The listing builds one solid part. Answer for the finished solid, in the listing's coordinates (mm). A direction names the side the tool comes from. Round coordinates to 2 decimals unless told otherwise and drop trailing zeros. Write each loop counter-clockwise with the first axis right and the second up, starting at its lowest first coordinate (ties: lowest second). Pieces come first, ordered by that corner, then holes. Notation, with made-up numbers: M 36,34 L 53,34 A32 ccw 53,61 Z; hole C 58,59.25 d6. An arc over 180 degrees is marked long. One line per item, written item: value. Start each with the question number.
(1) Given P1, Ø6, axis at x = 23, y = -94.5, coming from the +Z side; P2, Ø5, axis at x = 13, y = -127, coming from the -Z side, each flat-ended and moving along its own axis, determine where each tip first touches the part or whether it passes through.
(2) Section B-B (y = -90) is taken. Determine the outline of the cut face in (x, z).
(3) Section A-A (z = 14.25) is taken. State how many separate pieces and enclosed holes the cut face has, plus the area to 3 significant figures.
(4) For a pull along X with two mould halves and no side action, classify faces 4 (the flat face through (15, -129, 4.5)), 5 (the flat face through (80, -101, 10)), 6 (the flat face through (-1, -30, 10)) as released by +X, released by -X, zero draft, split by the parting line, or undercut.
(5) Consider probe 1 along Y at (x, z) = (20, 4.5); probe 2 along X at (y, z) = (-153, 14.75); probe 3 along Y at (x, z) = (-20, 17). Determine where each line is inside the solid, lowest interval first.
(6) Section C-C (x = -20) is taken. Determine the outline of the cut face in (y, z).
(7) For faces 1 (the flat face through (-1, -99, 20)), 2 (the flat face through (15, -155, 4.5)), 3 (the cylindrical face through (-15.386, -58.872, 13.591)), determine the directions among +Z, -Z, +X, -X, +Y, -Y from which every point of the face is accessible in a straight line to the end or side of a thin tool.
```python
from build123d import *

# Parameters (mm, degrees)
SKETCH1_W               = 160
SKETCH1_H               = 140
BOSS_EXTRUDE1_DEPTH     = 20
CUT_EXTRUDE1_DEPTH      = 189.944436277
CUT_EXTRUDE1_DEPTH_BACK = 189.944436277
SKETCH2_R               = 6.75
SKETCH3_R               = 10
CUT_EXTRUDE3_DEPTH      = 13
CUT_EXTRUDE4_DEPTH      = 189.944436277
CUT_EXTRUDE4_DEPTH_BACK = 189.944436277
SKETCH4_R               = 2.25
SKETCH5_R               = 4
CUT_EXTRUDE6_DEPTH      = 4.5


with BuildPart() as part:
    # Sketch1 → Boss-Extrude1 (new body)
    with BuildSketch(Plane.XY):
        with Locations((0, -100)):
            Rectangle(SKETCH1_W, SKETCH1_H)
    extrude(amount=BOSS_EXTRUDE1_DEPTH)

    # Sketch2 → Cut-Extrude1 (cut, two sides: drawn at the far end of the back side and taken through both)
    with BuildSketch(Plane.XY.offset(-CUT_EXTRUDE1_DEPTH_BACK)):
        with Locations((-20, -50)):
            Circle(SKETCH2_R)
        with Locations((-20, -90)):
            Circle(SKETCH2_R)
        with Locations((20, -50)):
            Circle(SKETCH2_R)
        with Locations((20, -90)):
            Circle(SKETCH2_R)
    extrude(amount=CUT_EXTRUDE1_DEPTH + CUT_EXTRUDE1_DEPTH_BACK, mode=Mode.SUBTRACT)

    # Sketch3 → Cut-Extrude3 (cut)
    with BuildSketch(Plane.XY.offset(20)):
        with Locations((-20, -50)):
            Circle(SKETCH3_R)
        with Locations((-20, -90)):
            Circle(SKETCH3_R)
        with Locations((20, -50)):
            Circle(SKETCH3_R)
        with Locations((20, -90)):
            Circle(SKETCH3_R)
    extrude(amount=-CUT_EXTRUDE3_DEPTH, mode=Mode.SUBTRACT)

    # Sketch4 → Cut-Extrude4 (cut, two sides: drawn at the far end of the back side and taken through both)
    with BuildSketch(Plane.XY.offset(-CUT_EXTRUDE4_DEPTH_BACK)):
        with Locations((-13, -127)):
            Circle(SKETCH4_R)
        with Locations((-13, -153)):
            Circle(SKETCH4_R)
        with Locations((13, -127)):
            Circle(SKETCH4_R)
        with Locations((13, -153)):
            Circle(SKETCH4_R)
    extrude(amount=CUT_EXTRUDE4_DEPTH + CUT_EXTRUDE4_DEPTH_BACK, mode=Mode.SUBTRACT)

    # Sketch5 → Cut-Extrude6 (cut)
    with BuildSketch(Plane.XY):
        with Locations((-13, -127)):
            Circle(SKETCH5_R)
        with Locations((-13, -153)):
            Circle(SKETCH5_R)
        with Locations((13, -127)):
            Circle(SKETCH5_R)
        with Locations((13, -153)):
            Circle(SKETCH5_R)
    extrude(amount=CUT_EXTRUDE6_DEPTH, mode=Mode.SUBTRACT)


solid = part.part
```
Recorded:
1. P1: stops at z = 7
1. P2: stops at z = 4.5
2. outline: M -80,0 L -26.75,0 L -26.75,7 L -30,7 L -30,20 L -80,20 Z; M -13.25,0 L 13.25,0 L 13.25,7 L 10,7 L 10,20 L -10,20 L -10,7 L -13.25,7 Z; M 26.75,0 L 80,0 L 80,20 L 30,20 L 30,7 L 26.75,7 Z
3. separate pieces: 1
3. enclosed holes: 8
3. area: 21,100 mm2
4. face 4: undercut
4. face 5: released by +X
4. face 6: zero draft
5. probe 1: y = -170 to -96.75, -83.25 to -56.75, -43.25 to -30
5. probe 2: x = -80 to -15.25, -10.75 to 10.75, 15.25 to 80
5. probe 3: y = -170 to -100, -80 to -60, -40 to -30
6. outline: M -170,0 L -96.75,0 L -96.75,7 L -100,7 L -100,20 L -170,20 Z; M -83.25,0 L -56.75,0 L -56.75,7 L -60,7 L -60,20 L -80,20 L -80,7 L -83.25,7 Z; M -43.25,0 L -30,0 L -30,20 L -40,20 L -40,7 L -43.25,7 Z
7. face 1: +Z, +X, -X, +Y, -Y
7. face 2: -Z
7. face 3: +Z
